Check sheet for the modelled part. Datum: model origin and axes. Units: mm. Face numbers are marked on the shaded views. A direction names the side the tool comes from. Round coordinates to 2 decimals unless told otherwise and drop trailing zeros. Loops run counter-clockwise (first coordinate to the right, second up) from the corner with the lowest first, then second, coordinate; pieces in that order, holes last. Notation, with made-up numbers: (48.5, -7) -> (83.5, -7) arc R31 ccw to (83.5, 30) -> close; hole circle Ø11 at (25, 60.5). An arc over 180 degrees is marked (long way). One line per item, written item: value. Start each with the question number.
1. Set-up check for the marked faces 1 and 2: record each of +Z, -Z, +X, -X, +Y, -Y from which the full face is reachable in a straight line by a thin tool's end or side.
2. Cross-section at D-D on y = 14.5. Record the cut outline in (x, z), then the cut area to 3 significant figures.
3. Release check for a two-part mould opening along X. For the marked faces 3, 4, 5 and 6 record: +X half, -X half, draft (parallel to the pull), parting line (faces both ways), or undercut.
4. Cross-section at C-C on x = 5. Record the cut outline in (y, z).
5. Go/stop test with flat-tipped pins: pin 1 (6 mm diameter, centred on x = 22, z = 6.5, fed in from +Y); pin 2 (1.5 mm diameter, centred on x = 12, z = 4.5, fed in from +Y); pin 3 (2 mm diameter, centred on x = 22.5, y = 18, fed in from +Z); pin 4 (2 mm diameter, centred on x = 14.5, y = 18.5, fed in from -Z). Record where each tip stops, or that it passes through.
6. Cross-section at B-B on y = 4. Record the cut outline in (x, z).
7. Cross-section at A-A on z = 5.5. Record the cut outline in (x, y).
8. Material ranges on L1, parallel to Y at x = 49.5, z = 9.25; L2, parallel to Y at x = 27, z = 14.25; L3, parallel to X at y = -9, z = 13, recorded low to high.
from build123d import *

# Parameters (mm, degrees)
F0_W     = 110.5350777507
F0_H     = 47.4778749049
F1_DEPTH = 15
F2_W     = 7.2117066011
F2_H     = 8.0962125212
F3_DEPTH = 110.5350777507
F4_T     = -2.5


with BuildPart() as f1:
    # F0 (on Top) → F1 (new body)
    with BuildSketch(Plane.XY):
        with Locations((-0.6117708981, -1.0488014668)):
            Rectangle(F0_W, F0_H)
    extrude(amount=F1_DEPTH)

    # F2 (on face) → F3 (cut, through all)
    with BuildSketch(Plane.YZ.offset(54.6557679772)):
        with Locations((19.0842826851, 4.0481062606)):
            Rectangle(F2_W, F2_H)
    extrude(amount=-F3_DEPTH, mode=Mode.SUBTRACT)

    # F4
    f4_openings = [f1.faces().sort_by_distance(p)[0] for p in [
        (-0.611771, -1.048801, 15),
    ]]
    offset(amount=F4_T, openings=f4_openings, kind=Kind.INTERSECTION)


solid = f1.part
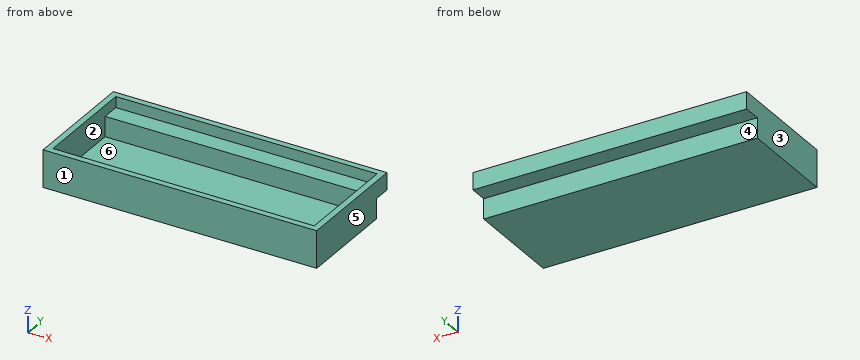
Taken from the geometry:
1. face 1: +Z, -Z, +X, -X, -Y
1. face 2: +Z
2. outline: (-55.88, 0) -> (54.66, 0) -> (54.66, 15) -> (52.16, 15) -> (52.16, 10.6) -> (-53.38, 10.6) -> (-53.38, 15) -> (-55.88, 15) -> close
2. area: 1,190 mm2
3. face 3: -X half
3. face 4: draft
3. face 5: +X half
3. face 6: undercut
4. outline: (-24.79, 0) -> (15.48, 0) -> (15.48, 8.1) -> (22.69, 8.1) -> (22.69, 15) -> (20.19, 15) -> (20.19, 10.6) -> (12.98, 10.6) -> (12.98, 2.5) -> (-22.29, 2.5) -> (-22.29, 15) -> (-24.79, 15) -> close
5. pin 1: stops at y = 22.69
5. pin 2: stops at y = 15.48
5. pin 3: stops at z = 10.6
5. pin 4: stops at z = 8.1
6. outline: (-55.88, 0) -> (54.66, 0) -> (54.66, 15) -> (52.16, 15) -> (52.16, 2.5) -> (-53.38, 2.5) -> (-53.38, 15) -> (-55.88, 15) -> close
7. outline: (-55.88, -24.79) -> (54.66, -24.79) -> (54.66, 15.48) -> (-55.88, 15.48) -> close; hole (-53.38, -22.29) -> (52.16, -22.29) -> (52.16, 12.98) -> (-53.38, 12.98) -> close
8. L1: y = -24.79 to -22.29, 12.98 to 22.69
8. L2: y = -24.79 to -22.29, 20.19 to 22.69
8. L3: x = -55.88 to -53.38, 52.16 to 54.66
